Can you work these out from the model? Positions are in its coordinate system, mm. Face numbers are marked on the shaded views. Coordinates: 2 decimals unless noted, no trailing zeros. Order: outer loops, then holes, each group sorted by start corner. A loop starts at its lowest first (then second) coordinate and runs counter-clockwise, first axis right, second up. Notation, with made-up numbers: (56.25, -25.5) - (102.25, -25.5) arc R10 cw to (102.25, -17.5) - close; hole circle Ø8 at (57, 87). An arc over 180 degrees is marked (long way). Return JSON: item names as keys, results as strings. Group by question number.
1) If we mould it in two halves opening along Y, with no side actions, what happens to the marked faces 1 and 2? For each: pulls with the +Y half, pulls with the -Y half, needs draft (parallel to the pull), parting line crosses it, or undercut.
2) If I drill on line 1 along Y through (x, z) = (0, 85); line 2 along X through (y, z) = (-94.5, 36.5); line 3 along X through (y, z) = (-96.5, 52), over which ranges is the centre line in solid material (lowest first)?
3) Imagine slicing it at A-A (x = 0). Write out the boundary of the cut face in (y, z).
4) Imagine slicing it at C-C (z = 176). Write out the boundary of the cut face in (x, y), and give its area (3 significant figures).
5) For pin 1 Ø4 at (x, y) = (108, -103.5) entering from +Z; pin 2 Ø10 at (y, z) = (-89, 36) entering from +X; pin 3 Ø6 at (x, y) = (-73, 130) entering from -Z, each with a flat end and sliding along its axis, tell me the tip position at first contact or that it passes through.
```python
from build123d import *

# Parameters (mm, degrees)
IZIM1_R                     = 180
Y_KSEKLIK_EKSTR_ZYON1_DEPTH = 200
RADYUS2_R                   = 10
IZIM2_R                     = 150
KES_EKSTR_ZYON1_DEPTH       = 200
RADYUS3_R                   = 5


with BuildPart() as part:
    # Çizim1 → Yükseklik-Ekstrüzyon1 (new body)
    with BuildSketch(Plane.XY):
        Circle(IZIM1_R)
    extrude(amount=Y_KSEKLIK_EKSTR_ZYON1_DEPTH)

    # Radyus2
    radyus2_edges = [part.edges().sort_by_distance(p)[0] for p in [
        (-180, 0, 0),
        (-180, 0, 200),
    ]]
    fillet(radyus2_edges, radius=RADYUS2_R)

    # Çizim2 → Kes-Ekstrüzyon1 (cut)
    with BuildSketch(Plane(origin=(0, 0, 0), x_dir=(-1, 0, 0), z_dir=(0, 0, -1))):
        Circle(IZIM2_R)
    extrude(amount=-KES_EKSTR_ZYON1_DEPTH, mode=Mode.SUBTRACT)

    # Radyus3
    radyus3_edges = [part.edges().sort_by_distance(p)[0] for p in [
        (150, 0, 200),
        (150, 0, 0),
    ]]
    fillet(radyus3_edges, radius=RADYUS3_R)


solid = part.part
```
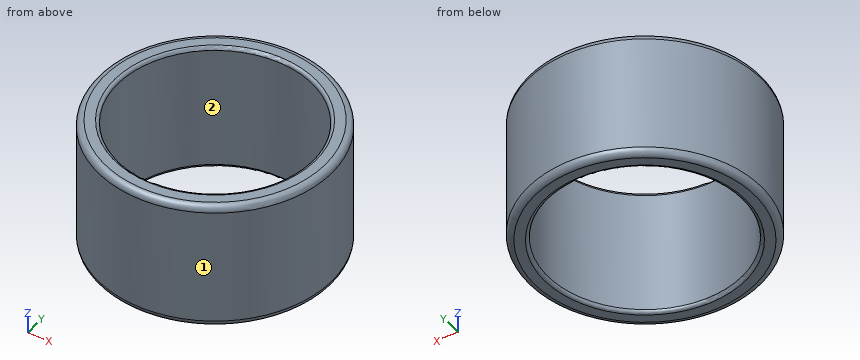
Calculated:
{
 "1": {"face 1": "parting line crosses it", "face 2": "undercut"},
 "2": {"line 1": "-180 to -150, 150 to 180", "line 2": "-153.2 to -116.49, 116.49 to 153.2", "line 3": "-151.95 to -114.84, 114.84 to 151.95"},
 "3": {"outline": "(-180, 10) arc R10 ccw to (-170, 0) - (-155, 0) arc R5 ccw to (-150, 5) - (-150, 195) arc R5 ccw to (-155, 200) - (-170, 200) arc R10 ccw to (-180, 190) - close; (150, 5) arc R5 ccw to (155, 0) - (170, 0) arc R10 ccw to (180, 10) - (180, 190) arc R10 ccw to (170, 200) - (155, 200) arc R5 ccw to (150, 195) - close"},
 "4": {"outline": "circle Ø360 at (0, 0); hole circle Ø300 at (0, 0)", "area": "31,100 mm2"},
 "5": {"pin 1": "z = 198.65", "pin 2": "x = 159.2", "pin 3": "z = 0.93"}
}
